Autodesk Fusion 360 part; units mm, degrees
sketch "Skizze1" plane through (0, 0, 0) normal (0, 0, 1) x (1, 0, 0)
  line L0 (-48.5045, 60.0252) -> (-48.5045, -50)
  line L1 (21.4307, 60.0126) -> (21.4307, -50)
  line L2 (-41.5077, 135.8568) -> (-13.5563, 144.0233)
  line L3 (-13.5563, 144.0233) -> (14.4793, 135.8568)
  line L4 (-41.4821, -125.8001) -> (-13.5254, -133.9377)
  line L5 (-13.5254, -133.9377) -> (14.4312, -125.8001)
  line L6 (14.4312, -125.8001) -> (14.4312, -57)
  line L7 (-41.4821, -125.8001) -> (-41.4821, -57)
  line L8 (-41.5077, 135.8568) -> (-41.5077, 66.6867)
  line L9 (14.4793, 135.8568) -> (14.4793, 66.6867)
  circle A0 centre (3.4202, 136.0177) radius 1.7651
  circle A1 centre (-30.4724, 136.0177) radius 1.7717
  circle A2 centre (-30.5621, -125.8912) radius 1.7405
  circle A3 centre (3.437, -125.8912) radius 1.7197
  circle A4 centre (-43.5796, -44.9629) radius 1.7343
  circle A5 centre (16.4191, -44.9629) radius 1.761
  circle A6 centre (-43.5796, 55.0289) radius 1.7075
  circle A7 centre (16.4191, 55.0289) radius 1.7507
  line L10 (21.4307, 60.0126) -> (21.4793, 60.0126)
  line L11 (14.4793, 67.0126) -> (14.4793, 66.6867)
  line L12 (-41.5077, 66.6867) -> (-41.5077, 67.0252)
  line L13 (-48.5077, 60.0252) -> (-48.5045, 60.0252)
  line L14 (-48.5045, -50) -> (-48.4821, -50)
  line L15 (21.4312, -50) -> (21.4307, -50)
  arc A8 (21.4312, -50) -> (14.4312, -57) centre (21.4312, -57) ccw
  arc A9 (-41.4821, -57) -> (-48.4821, -50) centre (-48.4821, -57) ccw
  arc A10 (-48.5077, 60.0252) -> (-41.5077, 67.0252) centre (-48.5077, 67.0252) ccw
  arc A11 (14.4793, 67.0126) -> (21.4793, 60.0126) centre (21.4793, 67.0126) ccw
  dimension "d1" = 7
  dimension "d2" = 7
  dimension "d3" = 7
  dimension "d4" = 7
extrude "Extrusion1" add sketch "Skizze1" along normal blind 3
sketch "Skizze2" plane through (0, 0, 0) normal (0, 0, 1) x (1, 0, 0)
  circle A0 centre (-13.6498, 118.1825) radius 1.7726
  circle A1 centre (-13.6498, 79.1243) radius 1.75
  circle A2 centre (-13.4454, 24.6727) radius 1.7602
  circle A3 centre (-13.5095, -14.2747) radius 1.7594
  circle A4 centre (-38.3105, 21.3875) radius 1.7537
  circle A5 centre (-38.3105, -36.6009) radius 1.7548
  circle A6 centre (11.0959, -36.6009) radius 1.7639
  circle A7 centre (11.0959, 21.3357) radius 1.7296
  circle A8 centre (-13.5725, -68.7537) radius 1.7556
  circle A9 centre (-13.5725, -107.7909) radius 1.7814
  dimension "d7" = 3.5
extrude "Extrusion2" cut sketch "Skizze2" along normal blind 10
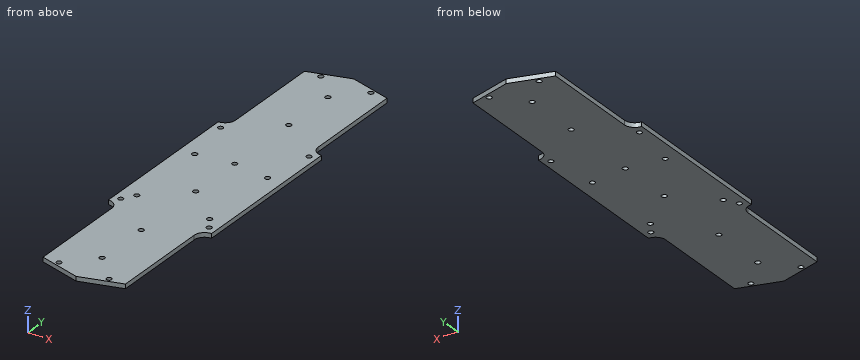
For this review, take the finished solid that the model builds, in its own axes (mm). Round coordinates to 2 decimals unless told otherwise and drop trailing zeros. Loops run counter-clockwise (first coordinate to the right, second up) from the corner with the lowest first, then second, coordinate; pieces in that order, holes last. Notation, with made-up numbers: (80, -13.75) - (103, -13.75) arc R26 cw to (103, 15.25) - close; hole circle Ø1 at (47.5, 24). An arc over 180 degrees is marked (long way). Put each result on its own line as item: value. Start each with the question number.
1. Consider section B-B on y = 107.5. State the section outline as (x, z) points, plus the area to 3 significant figures.
2. Consider section C-C on x = -4.5. State the section outline as (y, z) points.
3. For probe 1 along Y at (x, z) = (2.5, 2.4); probe 2 along Y at (x, z) = (-30, 0.2); probe 3 along X at (y, z) = (-91, 1.25), list the stretches that pass through material, from the lowest coordinate up. Write a range as [from, to].
4. Insertion check: P1, Ø4, axis at x = -30.56, y = -125.89, coming from the +Z side; P2, Ø0.9, axis at y = -108, z = 1.5, coming from the +X side; P3, Ø0.9, axis at y = 88, z = 1, coming from the -X side; P4, Ø1, axis at x = -28, z = 0.5, coming from the +Y side. Each pin has a flat end and moves straight along its axis. Give the tip position at first contact, or say it passes through.
5. Consider section A-A on z = 1.4. State how many separate pieces and enclosed holes the cut face has, plus the area to 3 significant figures.
Result sheet:
1. outline: (-41.51, 0) - (14.48, 0) - (14.48, 3) - (-41.51, 3) - close
1. area: 168 mm^2
2. outline: (-131.31, 0) - (141.39, 0) - (141.39, 3) - (-131.31, 3) - close
3. probe 1: [-129.27, -127.33], [-124.45, 134.51], [137.52, 139.35]
3. probe 2: [-129.14, -127.54], [-124.24, 134.31], [137.73, 139.22]
3. probe 3: [-41.48, 14.43]
4. P1: z = 3
4. P2: x = 14.43
4. P3: x = -41.51
4. P4: y = 139.95
5. separate pieces: 1
5. enclosed holes: 18
5. area: 16,500 mm^2
